Design review of the part built by this model. Coordinates are the model's own, in mm. A direction names the side the tool comes from. Round coordinates to 2 decimals unless told otherwise and drop trailing zeros. Order: outer loops, then holes, each group sorted by start corner. A loop starts at its lowest first (then second) coordinate and runs counter-clockwise, first axis right, second up. Notation, with made-up numbers: M -20,-4.5 L 7,-4.5 A29 ccw 7,28.5 Z; hole C 60,71.25 d4. An arc over 180 degrees is marked long. Write item = value, one per line. Start each with the question number.
```python
from build123d import *

# Parameters (mm, degrees)
F0_W     = 226.923436
F0_H     = 124.384374
F1_DEPTH = 127
F2_W     = 69.073379
F2_H     = 147.068739
F3_DEPTH = 50.8


with BuildPart() as f1:
    # F0 (on Front) → F1 (new body)
    with BuildSketch(Plane.XZ):
        Rectangle(F0_W, F0_H)
    extrude(amount=F1_DEPTH)

    # F2 (on face) → F3 (join)
    with BuildSketch(Plane.YZ.offset(113.461718)):
        with Locations((-2.807253, -3.165864)):
            Rectangle(F2_W, F2_H)
    extrude(amount=F3_DEPTH)


solid = f1.part
```
(1) Consider section D-D, the plane y = -95.5. Write out the cut boundary in (x, z).
(2) Consider section C-C, the plane x = -87.5. Write out the cut boundary in (y, z).
(3) Insertion check: pin 1 (5 mm diameter, centred on x = 132.5, z = -39, fed in from -Y); pin 2 (1.5 mm diameter, centred on x = 48.5, z = 50, fed in from +Y); pin 3 (4 mm diameter, centred on x = 56.5, y = -102, fed in from +Z). Each pin has a flat end and moves straight along its axis. Give the tip position at first contact, or say it passes through.
(4) Consider section B-B, the plane z = 1.5. Write out the cut boundary in (x, y).
(5) For line 1 along Y through (x, z) = (-75.5, 57); line 2 along Z through (x, y) = (47, -93.5); line 3 along X through (y, z) = (-49.5, 30), list the stretches that pass through material, from the lowest coordinate up. Write a range as [from, to].
(6) For faces 1 (the face through (-2, 0, 1)), 2 (the face through (139, -37.344, -4)), 3 (the face through (-2, -63, -62.192)), 4 (the face through (139, -3, 70.369)), 5 (the face through (-2, -63, 62.192)), list the 3-axis set-ups (+Z, -Z, +X, -X, +Y, -Y) from which the entire face can be reached by the end or side of a thin tool; tool diameter is ignored.
(7) Consider section A-A, the plane y = -28.5. Write out the cut boundary in (x, z), then the cut area to 3 significant figures.
Completed:
q1.outline = M -113.46,-62.19 L 113.46,-62.19 L 113.46,62.19 L -113.46,62.19 Z
q2.outline = M -127,-62.19 L 0,-62.19 L 0,62.19 L -127,62.19 Z
q3.pin_1 = -37.34
q3.pin_2 = 0
q3.pin_3 = 62.19
q4.outline = M -113.46,-127 L 113.46,-127 L 113.46,-37.34 L 164.26,-37.34 L 164.26,31.73 L 113.46,31.73 L 113.46,0 L -113.46,0 Z
q5.line_1 = [-127, 0]
q5.line_2 = [-62.19, 62.19]
q5.line_3 = [-113.46, 113.46]
q6.face_1 = +Z, -Z, -X, +Y
q6.face_2 = +Z, -Z, +X, -Y
q6.face_3 = -Z, -X, +Y, -Y
q6.face_4 = +Z, +X, -X, +Y, -Y
q6.face_5 = +Z, -X, +Y, -Y
q7.outline = M -113.46,-62.19 L 113.46,-62.19 L 113.46,-76.7 L 164.26,-76.7 L 164.26,70.37 L 113.46,70.37 L 113.46,62.19 L -113.46,62.19 Z
q7.area = 35,700 mm2
